The listing builds one solid part. Answer for the finished solid, in the listing's coordinates (mm). Give positions to 0.01 mm unless a question says otherwise; leave off trailing zeros. Answer in a Markdown table with one row per item. Add a question column.
```python
from build123d import *

# Parameters (mm, degrees)
F4_R     = 4.7625
F4_R_2   = 3.5179
F5_DEPTH = 330.2


with BuildPart() as f5:
    # F4 (on 3pt) → F5 (new body)
    with BuildSketch(Plane(origin=(-45.2213167265, -18.9210530236, 0), x_dir=(0.3859853229, -0.9225049217, 0), z_dir=(-0.9225049217, -0.3859853229, 0))):
        with Locations((117.1581250533, 0)):
            Circle(F4_R)
        with Locations((117.1581250533, 0)):
            Circle(F4_R_2, mode=Mode.SUBTRACT)
    extrude(amount=-F5_DEPTH)

    # F6: F5 across plane


with BuildPart() as f5_1:
    add(f5.part)
    add(f5.part.mirror(Plane.XZ))


solid = f5_1.part
```
(1) Find the intervals of material crossed by line 1 along Y through (x, z) = (101.5, -2); line 2 along Y through (x, z) = (124, 1); line 3 along X through (y, z) = (-22, -0.25), in increasing order. Write a range as [from, to].
(2) The mould has two halves that part along Y. Classify faces 1 (the face through (0, 127, -4)), 2 (the face through (0, -127, -4)), 3 (the face through (148.82, -60.93, 3.22)): pulls with the +Y half, pulls with the -Y half, needs draft (parallel to the pull), parting line crosses it, or undercut.
(3) Given pin 1 Ø3 at (y, z) = (-31.5, -1) entering from -X; pin 2 Ø3 at (x, z) = (101, 0.5) entering from +Y; pin 3 Ø3 at (x, y) = (138.5, -71.5) entering from +Z, each flat-ended and moving along its own axis, determine where each tip first touches the part or whether it passes through.
(4) A cutting plane is placed at A-A on x = 31.5. Give the number of separate pieces and of enclosed holes in the cut face, plus the area to 3 significant figures.
Evaluation:
| question | item | result |
|---|---|---|
| 1 | line 1 | y = [-89.22, -87.67], [-81.39, -79.85], [79.85, 81.39], [87.67, 89.22] |
| 1 | line 2 | y = [-80.16, -78.77], [-71.46, -70.07], [70.07, 71.46], [78.77, 80.16] |
| 1 | line 3 | x = [238.63, 241.86], [260.04, 263.27] |
| 2 | face 1 | pulls with the +Y half |
| 2 | face 2 | pulls with the -Y half |
| 2 | face 3 | undercut |
| 3 | pin 1 | stops at x = 212.53 |
| 3 | pin 2 | stops at y = 90.52 |
| 3 | pin 3 | stops at z = 4.7 |
| 4 | separate pieces | 2 |
| 4 | enclosed holes | 2 |
| 4 | area | 70.2 mm² |
